Verification items for this drawing (mm, ordinates from the low corner). Give positions to 0.01 mm unless a question says otherwise; leave off trailing zeros. Order: outer loops, then holes, each group sorted by start corner. A loop starts at its lowest first (then second) coordinate and runs counter-clockwise, first axis right, second up.
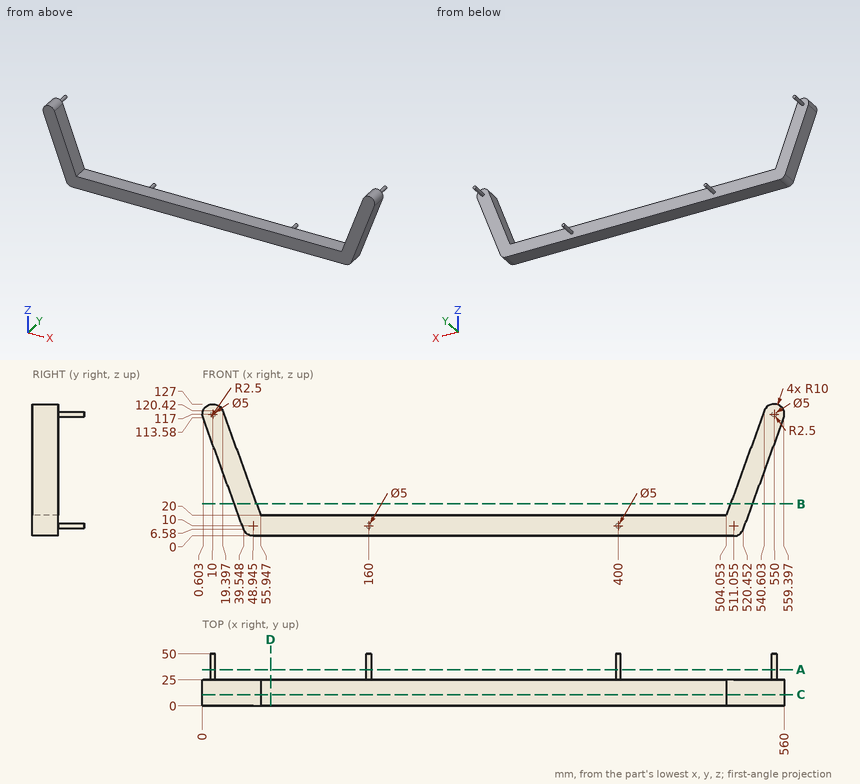
Q1. Cross-section at B-B, the plane z = 31. Record the boundary of the cut face in (x, y), and give its area (3 significant figures).
Q2. Cross-section at C-C, the plane y = 11. Record the boundary of the cut face in (x, z) (1 decimal).
Q3. Gauge pin test, flat ends, axial feed: P1, Ø7.5, axis at x = 194, y = 7.5, coming from the +Z side; P2, Ø12, axis at y = 25, z = 56.5, coming from the -X side (1 decimal); P3, Ø1, axis at y = 8.5, z = 101.5, coming from the +X side. Record the tip position at first contact, or that the pin passes through.
Q4. Thickness scan on L1, parallel to Z at x = 175, y = 19; L2, parallel to Y at x = 166, z = 13.5; L3, parallel to X at y = 15.5, z = 92.5 (1 decimal). Record the ranges inside material, lowest first.
Q5. Cross-section at D-D, the plane x = 65.5. Record the boundary of the cut face in (y, z).
Q6. Cross-section at A-A, the plane y = 35. Record the boundary of the cut face in (x, z) (1 decimal).
Answers follow:
1. outline: (30.66, 0) - (51.94, 0) - (51.94, 25) - (30.66, 25) - close; (508.06, 0) - (529.34, 0) - (529.34, 25) - (508.06, 25) - close
1. area: 1,060 mm2
2. outline: (0.6, 113.6) - (39.5, 6.6) arc R10 ccw to (48.9, 0) - (511.1, 0) arc R10 ccw to (520.5, 6.6) - (559.4, 113.6) arc R10 ccw to (540.6, 120.4) - (504.1, 20) - (55.9, 20) - (19.4, 120.4) arc R10 ccw to start
3. P1: stops at z = 20
3. P2: stops at x = 19.2
3. P3: stops at x = 555.18
4. L1: z = 0 to 20
4. L2: y = 0 to 25
4. L3: x = 8.3 to 29.6, 530.4 to 551.7
5. outline: (0, 0) - (25, 0) - (25, 20) - (0, 20) - close
6. outline: circle Ø5 at (10, 117); circle Ø5 at (160, 10); circle Ø5 at (400, 10); circle Ø5 at (550, 117)
